from build123d import *

# Parameters (mm, degrees)
ESQUISSE1_W        = 40.4
ESQUISSE1_H        = 20
ESQUISSE1_W_2      = 38.4
ESQUISSE1_H_2      = 18
BOSS_EXTRU_1_DEPTH = 21
CONG_1_R           = 1


with BuildPart() as part:
    # Esquisse1 → Boss.-Extru.1 (new body)
    with BuildSketch(Plane(origin=(0, 0, 0), x_dir=(1, 0, 0), z_dir=(0, 1, 0))):
        with Locations((-8.710891089, 0)):
            Rectangle(ESQUISSE1_W, ESQUISSE1_H)
        with Locations((-8.710891089, 0)):
            Rectangle(ESQUISSE1_W_2, ESQUISSE1_H_2, mode=Mode.SUBTRACT)
    extrude(amount=BOSS_EXTRU_1_DEPTH)

    # Congé1
    cong_1_edges = [part.edges().sort_by_distance(p)[0] for p in [
        (-28.910891089, 10.5, -10),
        (11.489108911, 10.5, -10),
        (11.489108911, 10.5, 10),
        (-28.910891089, 10.5, 10),
    ]]
    fillet(cong_1_edges, radius=CONG_1_R)


solid = part.part
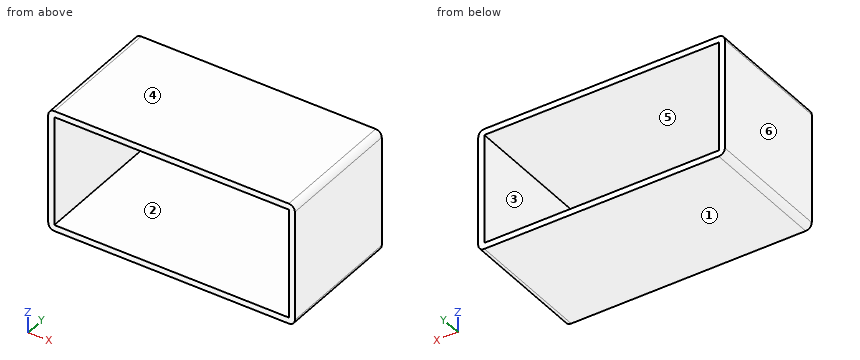
Here's how the part is built. I have some questions about the finished solid (model axes, mm). Face numbers are marked on the shaded views. A direction names the side the tool comes from. Round coordinates to 2 decimals unless told otherwise and drop trailing zeros. Loops run counter-clockwise (first coordinate to the right, second up) from the corner with the lowest first, then second, coordinate; pieces in that order, holes last. Notation, with made-up numbers: (55, 82) - (105, 82) arc R19 ccw to (105, 106) - close; hole circle Ø10 at (-1.75, 34.5). An arc over 180 degrees is marked (long way). One line per question, with ' | ' between items. Start each with the question number.
Q1. I want a section at C-C (y = 10.5). Write out the boundary of the cut face in (x, z).
Q2. I want a section at A-A (x = -7.5). Write out the boundary of the cut face in (y, z).
Q3. Please list where these lines run through material, in increasing order: line 1 (X direction, y = 1, z = 1); line 2 (Z direction, x = -24, y = 2). Write a range as [from, to].
Q4. For the marked faces 1 and 2, which set-ups out of +Z, -Z, +X, -X, +Y, -Y let a thin tool reach every point of the face, with its end or its side?
Q5. I want a section at B-B (z = -5.25). Write out the boundary of the cut face in (x, y), then the cut area to 3 significant figures.
Q6. We'd pull the mould along Z, two halves only. Please class the marked faces 3, 4, 5 and 6: +Z half, -Z half, draft (parallel to the pull), parting line (faces both ways), or undercut.
Response values:
1) outline: (-28.91, -9) arc R1 ccw to (-27.91, -10) - (10.49, -10) arc R1 ccw to (11.49, -9) - (11.49, 9) arc R1 ccw to (10.49, 10) - (-27.91, 10) arc R1 ccw to (-28.91, 9) - close; hole (-27.91, -9) - (10.49, -9) - (10.49, 9) - (-27.91, 9) - close
2) outline: (0, -10) - (21, -10) - (21, -9) - (0, -9) - close; (0, 9) - (21, 9) - (21, 10) - (0, 10) - close
3) line 1: x = [-28.91, -27.91], [10.49, 11.49] | line 2: z = [-10, -9], [9, 10]
4) face 1: -Z, +X, -X, +Y, -Y | face 2: +Y, -Y
5) outline: (-28.91, 0) - (-27.91, 0) - (-27.91, 21) - (-28.91, 21) - close; (10.49, 0) - (11.49, 0) - (11.49, 21) - (10.49, 21) - close | area: 42.0 mm²
6) face 3: undercut | face 4: +Z half | face 5: undercut | face 6: draft
